For this review, take the finished solid that the model builds, in its own axes (mm). A direction names the side the tool comes from. Give positions to 0.01 mm unless a question says otherwise; leave off trailing zeros. Loops run counter-clockwise (first coordinate to the right, second up) from the corner with the lowest first, then second, coordinate; pieces in that order, holes last.
Autodesk Inventor part; units mm, degrees
ref_plane "to_b_XY" through (0, 14.2748, 0) normal (0, 0, -1) x (1, 0, 0)
ref_plane "to_b_YZ" through (0, 14.2748, 0) normal (1, 0, 0) x (0, -1, 0)
ref_plane "to_b_ZX" through (0, 14.2748, 0) normal (0, -1, 0) x (0, 0, -1)
sketch "Sketch_1" plane through (0, 0, 0) normal (0, 1, 0) x (-1, 0, 0)
  arc A0 (37, 16) -> (33, 20) centre (33, 16) ccw
  line L0 (33, 20) -> (0.6018, 20)
  line L1 (0.6018, 20) -> (0.6018, -20)
  line L2 (0.6018, -20) -> (33, -20)
  arc A1 (33, -20) -> (37, -16) centre (33, -16) ccw
  line L3 (37, -16) -> (37, 16)
  circle A2 centre (22.5, 10.5) radius 4.1
  circle A3 centre (22.5, -10.5) radius 4.1
extrude "Extrusion1" add sketch "Sketch_1" along normal blind 7.9248
sketch "Sketch_2" plane through (0, 0, 0) normal (0, 0, 1) x (1, 0, 0)
  line L0 (-74, 15.8496) -> (-74, -7.9248)
  line L1 (-74, -7.9248) -> (37, -7.9248)
  line L2 (37, -7.9248) -> (37, 15.8496)
  line L3 (37, 15.8496) -> (-74, 15.8496)
  arc A0 (-37, 0.5) -> (-36.5, 0) centre (-36.5, 0.5) ccw
  line L4 (-36.5, 0) -> (-0.6, 0)
  line L5 (-0.6, 0) -> (-0.6, 7.9248)
  line L6 (-0.6, 7.9248) -> (-35.5, 7.9248)
  arc A1 (-35.5, 7.9248) -> (-37, 6.4248) centre (-35.5, 6.4248) ccw
  line L7 (-37, 6.4248) -> (-37, 0.5)
extrude "Extrusion2" cut sketch "Sketch_2" along normal mid plane 40
sketch "Sketch_3" plane through (0, 0, 0) normal (1, 0, 0) x (0, 1, 0)
  line L0 (15.8496, 40) -> (-7.9248, 40)
  line L1 (-7.9248, 40) -> (-7.9248, -40)
  line L2 (-7.9248, -40) -> (15.8496, -40)
  line L3 (15.8496, -40) -> (15.8496, 40)
  arc A0 (0.5, 20) -> (0, 19.5) centre (0.5, 19.5) ccw
  line L4 (0, 19.5) -> (0, -19.5)
  arc A1 (0, -19.5) -> (0.5, -20) centre (0.5, -19.5) ccw
  line L5 (0.5, -20) -> (6.4248, -20)
  arc A2 (6.4248, -20) -> (7.9248, -18.5) centre (6.4248, -18.5) ccw
  line L6 (7.9248, -18.5) -> (7.9248, 18.5)
  arc A3 (7.9248, 18.5) -> (6.4248, 20) centre (6.4248, 18.5) ccw
  line L7 (6.4248, 20) -> (0.5, 20)
extrude "Extrusion3" cut sketch "Sketch_3" against normal blind 74
sketch "Sketch_4" plane through (0, 0, 0) normal (0, 0, 1) x (1, 0, 0)
  circle A0 centre (0, 14.2748) radius 10.5
extrude "Extrusion4" cut sketch "Sketch_4" along normal mid plane 40
sketch "Sketch_5" plane through (0, 14.2748, 0) normal (0, 1, 0) x (1, 0, 0)
  arc A0 (-9.9568, -11.5) -> (-9.4568, -12) centre (-9.4568, -11.5) ccw
  line L0 (-9.4568, -12) -> (-0.6018, -12)
  line L1 (-0.6018, -12) -> (-0.6018, -1)
  line L2 (-0.6018, -1) -> (-9.4568, -1)
  arc A1 (-9.4568, -1) -> (-9.9568, -1.5) centre (-9.4568, -1.5) ccw
  line L3 (-9.9568, -1.5) -> (-9.9568, -11.5)
extrude "Extrusion5" add sketch "Sketch_5" against normal blind 11.7348
sketch "Sketch_6" plane through (0, 14.2748, 0) normal (0, 1, 0) x (1, 0, 0)
  line L0 (0, -1) -> (0, -12)
  line L1 (0, -12) -> (-9.4568, -12)
  arc A0 (-9.9568, -11.5) -> (-9.4568, -12) centre (-9.4568, -11.5) ccw
  line L2 (-9.9568, -11.5) -> (-9.9568, -1.5)
  arc A1 (-9.4568, -1) -> (-9.9568, -1.5) centre (-9.4568, -1.5) ccw
  line L3 (-9.4568, -1) -> (0, -1)
  line L4 (0, -1) -> (0, -12)
revolve "Revolution1" add sketch "Sketch_6" angle 360 about axis through (0, 14.2748, 1) along (0, 0, -1)
sketch "Sketch_7" plane through (0, 14.2748, 0) normal (0, 1, 0) x (1, 0, 0)
  arc A0 (-9.9568, 14.5) -> (-9.4568, 14) centre (-9.4568, 14.5) ccw
  line L0 (-9.4568, 14) -> (-0.6018, 14)
  line L1 (-0.6018, 14) -> (-0.6018, 20)
  line L2 (-0.6018, 20) -> (-9.4568, 20)
  arc A1 (-9.4568, 20) -> (-9.9568, 19.5) centre (-9.4568, 19.5) ccw
  line L3 (-9.9568, 19.5) -> (-9.9568, 14.5)
extrude "Extrusion6" add sketch "Sketch_7" against normal blind 11.7348
sketch "Sketch_8" plane through (0, 14.2748, 0) normal (0, 1, 0) x (1, 0, 0)
  line L0 (0, 20) -> (0, 14)
  line L1 (0, 14) -> (-9.4568, 14)
  arc A0 (-9.9568, 14.5) -> (-9.4568, 14) centre (-9.4568, 14.5) ccw
  line L2 (-9.9568, 14.5) -> (-9.9568, 19.5)
  arc A1 (-9.4568, 20) -> (-9.9568, 19.5) centre (-9.4568, 19.5) ccw
  line L3 (-9.4568, 20) -> (0, 20)
  line L4 (0, 20) -> (0, 14)
revolve "Revolution2" add sketch "Sketch_8" angle 360 about axis through (0, 14.2748, -20) along (0, 0, -1)
sketch "Sketch_9" plane through (0, 0, 0) normal (0, 0, 1) x (1, 0, 0)
  circle A0 centre (0, 14.2748) radius 4.25
extrude "Extrusion7" cut sketch "Sketch_9" along normal mid plane 40
ref_plane "to_b_XY" through (0, 14.2748, 0) normal (0, 0, -1) x (1, 0, 0)
ref_plane "to_b_YZ" through (0, 14.2748, 0) normal (1, 0, 0) x (0, -1, 0)
ref_plane "to_b_ZX" through (0, 14.2748, 0) normal (0, -1, 0) x (0, 0, -1)
ref_plane "to_pin_XY" through (0, 14.2748, 0) normal (0, 0, 1) x (1, 0, 0)
ref_plane "to_pin_YZ" through (0, 14.2748, 0) normal (1, 0, 0) x (0, 1, 0)
ref_plane "to_pin_ZX" through (0, 14.2748, 0) normal (0, 1, 0) x (0, 0, 1)
ref_plane "to_washer1_XY" through (0, 14.2748, 12.1745) normal (0, 0, -1) x (1, 0, 0)
ref_plane "to_washer1_YZ" through (0, 14.2748, 12.1745) normal (1, 0, 0) x (0, -1, 0)
ref_plane "to_washer1_ZX" through (0, 14.2748, 12.1745) normal (0, -1, 0) x (0, 0, -1)
ref_plane "to_washer2_XY" through (0, 14.2748, 0.8255) normal (0, 0, 1) x (1, 0, 0)
ref_plane "to_washer2_YZ" through (0, 14.2748, 0.8255) normal (1, 0, 0) x (0, 1, 0)
ref_plane "to_washer2_ZX" through (0, 14.2748, 0.8255) normal (0, 1, 0) x (0, 0, 1)
ref_plane "to_washer3_XY" through (0, 14.2748, -13.8255) normal (0, 0, -1) x (1, 0, 0)
ref_plane "to_washer3_YZ" through (0, 14.2748, -13.8255) normal (1, 0, 0) x (0, -1, 0)
ref_plane "to_washer3_ZX" through (0, 14.2748, -13.8255) normal (0, -1, 0) x (0, 0, -1)
properties part number "4489_a"
Q1. Consider section C-C on y = 3.25. Give the boundary of the cut face in (x, z).
Answers:
outline: (-37, -16) arc R4 ccw to (-33, -20) - (-0.6, -20) - (-0.6, 20) - (-33, 20) arc R4 ccw to (-37, 16) - close; hole circle Ø8.2 at (-22.5, -10.5); hole circle Ø8.2 at (-22.5, 10.5)
Q2. Consider section A-A on x = -22.5. Give the boundary of the cut face in (y, z).
Answers:
outline: (0, -19.5) arc R0.5 ccw to (0.5, -20) - (6.42, -20) arc R1.5 ccw to (7.92, -18.5) - (7.92, -14.6) - (0, -14.6) - close; (0, -6.4) - (7.92, -6.4) - (7.92, 6.4) - (0, 6.4) - close; (0, 14.6) - (7.92, 14.6) - (7.92, 18.5) arc R1.5 ccw to (6.42, 20) - (0.5, 20) arc R0.5 ccw to (0, 19.5) - close
Q3. Mouldability with a two-part tool opening along Y and no side actions: class faces 1 (the cylindrical face through (-4.879, 4.977, -6.605)), 2 (the cylindrical face through (4.054, 15.551, -16.958)), 3 (the flat face through (-17, 3, 20)) as +Y half, -Y half, draft (parallel to the pull), parting line (faces both ways), or undercut.
Answers:
face 1: +Y half
face 2: undercut
face 3: draft
Q4. Machinability: for faces 4 (the flat face through (-4.1, 16.1, 1)), 5 (the cylindrical face through (-22.458, 7.474, -19.572)), 6 (the flat face through (0, 9, 12)), which of the approach directions +Z, -Z, +X, -X, +Y, -Y give a long, thin tool a straight path to every point of the face, cutting with its end or side? Answer none if there is none.
Answers:
face 4: +X, +Y
face 5: -Z, -X, +Y
face 6: +Z, +X, +Y
Q5. Consider section B-B on z = -10.5. Give the boundary of the cut face in (x, y).
Answers:
outline: (-37, 0.5) arc R0.5 ccw to (-36.5, 0) - (-26.6, 0) - (-26.6, 7.92) - (-35.5, 7.92) arc R1.5 ccw to (-37, 6.42) - close; (-18.4, 0) - (-0.6, 0) - (-0.6, 3.79) arc R10.5 cw to (-8.36, 7.92) - (-18.4, 7.92) - close
Q6. For probe 1 along Z at (x, y) = (-22.5, 5); probe 2 along Y at (x, z) = (0, 4); probe 3 along Z at (x, y) = (-3, 21.25), list the stretches that pass through material, from the lowest coordinate up.
Answers:
probe 1: z = -20 to -14.6, -6.4 to 6.4, 14.6 to 20
probe 2: y = 4.32 to 10.02, 18.52 to 24.23
probe 3: z = -20 to -14, 1 to 12
Q7. Consider section D-D on z = -3. Give the boundary of the cut face in (x, y), plus the area to 3 significant figures.
Answers:
outline: (-37, 0.5) arc R0.5 ccw to (-36.5, 0) - (-0.6, 0) - (-0.6, 3.79) arc R10.5 cw to (-8.36, 7.92) - (-35.5, 7.92) arc R1.5 ccw to (-37, 6.42) - close
area: 266 mm2
Q8. For pin 1 Ø10 at (y, z) = (15, 5.5) entering from -X; pin 2 Ø10 at (y, z) = (15.5, -11.5) entering from +X; pin 3 Ø6 at (x, z) = (-3, -5.5) entering from +Y; pin 4 Ø5.5 at (y, z) = (3.5, -4.5) entering from +X, all flat-tipped, find the tip position at first contact; note any pin that passes through.
Answers:
pin 1: stops at x = -9.96
pin 2: stops at x = 9.96
pin 3: stops at y = 5.66
pin 4: stops at x = -0.6
